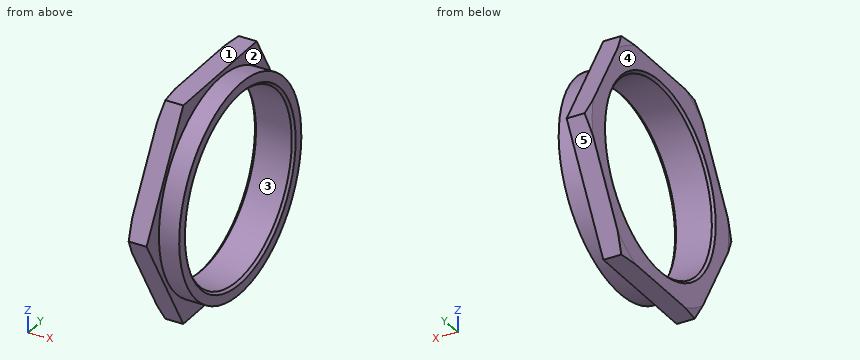
```python
from build123d import *

# Parameters (mm, degrees)
CHAMFER1_SIZE  = 0.5
CHAMFER1_SIZE2 = 1.866025404
SKETCH2_R      = 30.350258036
EXTRUDE1_DEPTH = 38.992630864
CHAMFER2_SIZE  = 0.5


with BuildPart() as part:
    # Sketch1 → Revolve1 (revolve)
    with BuildSketch(Plane.XY, mode=Mode.PRIVATE) as revolve1_sk:
        Polygon((0, 19.25), (0, 26.2), (4.2, 26.2), (4.2, 21.8), (8.4, 21.8), (8.4, 19.25), align=None)
    revolve(revolve1_sk.sketch.rotate(Axis((0, 0, 0), (1, 0, 0)), 90), axis=Axis((0, 0, 0), (1, 0, 0)))

    # Chamfer1
    chamfer1_edges = [part.edges().sort_by_distance(p)[0] for p in [
        (0, 0, -26.2),
    ]]
    chamfer1_side = [part.faces().sort_by_distance(p)[0] for p in [
        (2.1, 0, -26.2),
    ]]
    chamfer(chamfer1_edges, length=CHAMFER1_SIZE, length2=CHAMFER1_SIZE2, reference=chamfer1_side[0])

    # Sketch2 → Extrude1 (cut, through all)
    with BuildSketch(Plane.ZY):
        Circle(SKETCH2_R)
        Polygon((0, 26.2), (-22.689865579, 13.1), (-22.689865579, -13.1), (0, -26.2), (22.689865579, -13.1), (22.689865579, 13.1), align=None, mode=Mode.SUBTRACT)
    extrude(amount=-EXTRUDE1_DEPTH, mode=Mode.SUBTRACT)

    # Chamfer2
    chamfer2_edges = [part.edges().sort_by_distance(p)[0] for p in [
        (8.4, 0, -19.25),
        (0, 0, -19.25),
    ]]
    chamfer(chamfer2_edges, length=CHAMFER2_SIZE)


solid = part.part
```
Check sheet for the modelled part. Datum: model origin and axes. Units: mm. Face numbers are marked on the shaded views. A direction names the side the tool comes from. Coordinates: 2 decimals unless noted, no trailing zeros. Write each loop counter-clockwise with the first axis right and the second up, starting at its lowest first coordinate (ties: lowest second). Pieces come first, ordered by that corner, then holes. Notation, with made-up numbers: M 88,47.5 L 125,47.5 A27 cw 125,68.5 Z; hole C 17,29.25 d6. An arc over 180 degrees is marked long. Use one line per item in the form item = value.
Item 1: Gauge pin test, flat ends, axial feed: pin 1 Ø1 at (x, y) = (6.5, -15.5) entering from -Z; pin 2 Ø1 at (x, z) = (1, -4) entering from +Y; pin 3 Ø13.5 at (y, z) = (1, -8) entering from +X; pin 4 Ø1.5 at (x, z) = (7, 5) entering from +Y. Record the tip position at first contact, or that the pin passes through.
Answer below:
pin_1 = -15.82
pin_2 = 24.18
pin_3 = through
pin_4 = 21.38
Item 2: Material ranges on L1, parallel to Y at x = 5, z = 0; L2, parallel to Y at x = 3, z = 0; L3, parallel to Z at x = 5, y = 3.5, recorded low to high. Write a range as from..to.
Answer below:
L1 = -21.8..-19.25, 19.25..21.8
L2 = -26.2..-19.25, 19.25..26.2
L3 = -21.52..-18.93, 18.93..21.52
Item 3: Set-up check for the marked faces 1 and 2: record each of +Z, -Z, +X, -X, +Y, -Y from which the full face is reachable in a straight line by a thin tool's end or side.
Answer below:
face_1 = +Z, +X, -X, +Y, -Y
face_2 = +X
Item 4: Release check for a two-part mould opening along Z. For the marked faces 3, 4 and 5 record: pulls with the +Z half, pulls with the -Z half, needs draft (parallel to the pull), parting line crosses it, or undercut.
Answer below:
face_3 = undercut
face_4 = needs draft
face_5 = pulls with the -Z half
Item 5: Sectioned sample at C-C, the plane y = -20.5. Record the cut outline in (x, z).
Answer below:
outline = M 0,-9.87 L 4.2,-9.87 L 4.2,-7.42 L 8.4,-7.42 L 8.4,7.42 L 4.2,7.42 L 4.2,9.87 L 0,9.87 Z
Item 6: Sectioned sample at A-A, the plane y = 0. Record the cut outline in (x, z).
Answer below:
outline = M 0,-22.69 L 4.2,-22.69 L 4.2,-21.8 L 8.4,-21.8 L 8.4,-19.75 L 7.9,-19.25 L 0.5,-19.25 L 0,-19.75 Z; M 0,19.75 L 0.5,19.25 L 7.9,19.25 L 8.4,19.75 L 8.4,21.8 L 4.2,21.8 L 4.2,22.69 L 0,22.69 Z
Item 7: Sectioned sample at B-B, the plane x = 2.5. Record the cut outline in (y, z), and give its area (3 significant figures).
Answer below:
outline = M -26.2,0 L -13.1,-22.69 L 13.1,-22.69 L 26.2,0 L 13.1,22.69 L -13.1,22.69 Z; hole C 0,0 d38.5
area = 619 mm^2
Item 8: Sectioned sample at D-D, the plane x = 6. Record the cut outline in (y, z), and give its area (3 significant figures).
Answer below:
outline = C 0,0 d43.6; hole C 0,0 d38.5
area = 329 mm^2
